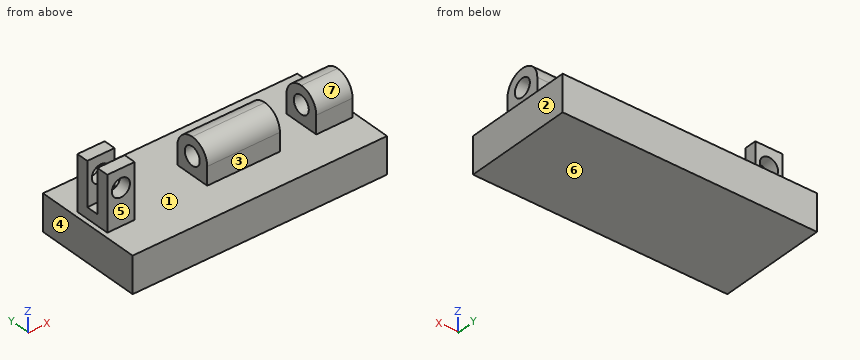
```python
from build123d import *

# Parameters (mm, degrees)
F0_W      = 177.8
F0_H      = 76.2
F1_DEPTH  = 25.4
F2_W      = 19.05
F2_H      = 38.1
F2_W_2    = 50.8
F2_H_2    = 25.4
F2_W_3    = 25.4
F3_DEPTH  = 25.4
F4_R      = 6.35
F5_DEPTH  = 101.6
F6_R      = 12.69999
F7_W      = 8.636
F7_H      = 30.48
F8_DEPTH  = 25.4
F9_R      = 6.35
F10_DEPTH = 25.4


# Not quite as in the source:
# - a fillet or chamfer is up to 0.001 mm smaller than in the source, because OpenCascade refuses the exact size


with BuildPart() as f1:
    # F0 (on Top) → F1 (new body)
    with BuildSketch(Plane.XY):
        with Locations((0, -12.7)):
            Rectangle(F0_W, F0_H)
    extrude(amount=F1_DEPTH)

    # F2 (on Front) → F3 (join)
    with BuildSketch(Plane.XZ):
        with Locations((-76.2, 44.45)):
            Rectangle(F2_W, F2_H)
        with Locations((9.525, 38.1)):
            Rectangle(F2_W_2, F2_H_2)
        with Locations((73.025, 38.1)):
            Rectangle(F2_W_3, F2_H_2)
    extrude(amount=F3_DEPTH)

    # F4 (on face) → F5 (cut, through all)
    with BuildSketch(Plane.YZ.offset(85.725)):
        with Locations((-12.7, 38.1)):
            Circle(F4_R)
    extrude(amount=-F5_DEPTH, mode=Mode.SUBTRACT)

    # F6 (radius 12.7 in the source; OpenCascade refuses exactly that, so slightly less here)
    f6_edges = [f1.edges().sort_by_distance(p)[0] for p in [
        (9.525, -25.4, 50.8),
        (9.525, 0, 50.8),
        (73.025, -25.4, 50.8),
        (73.025, 0, 50.8),
    ]]
    fillet(f6_edges, radius=F6_R)

    # F7 (on face) → F8 (cut)
    with BuildSketch(Plane(origin=(-85.725, 0, 0), x_dir=(0, -1, 0), z_dir=(-1, 0, 0))):
        with Locations((12.7, 48.26)):
            Rectangle(F7_W, F7_H)
    extrude(amount=-F8_DEPTH, mode=Mode.SUBTRACT)

    # F9 (on face) → F10 (cut)
    with BuildSketch(Plane.XZ.offset(25.4)):
        with Locations((-76.2, 50.8)):
            Circle(F9_R)
    extrude(amount=-F10_DEPTH, mode=Mode.SUBTRACT)


solid = f1.part
```
Geometry check sheet. Reference: the model listing, model coordinates, mm. Face numbers are marked on the shaded views. A direction names the side the tool comes from. Coordinates: 2 decimals unless noted, no trailing zeros. Order: outer loops, then holes, each group sorted by start corner. A loop starts at its lowest first (then second) coordinate and runs counter-clockwise, first axis right, second up. Notation, with made-up numbers: (-26.75, 51.25) - (16.25, 51.25) arc R19 cw to (16.25, 83.25) - close; hole circle Ø5 at (38.5, 88). An arc over 180 degrees is marked (long way). Answer as a JSON object with one key per item and string values. Group by question number.
Item 1: Sectioned sample at C-C, the plane y = -3.5. Record the cut outline in (x, z) (3 decimals), and give its area (3 significant figures).
Item 2: Sectioned sample at D-D, the plane z = 35. Record the cut outline in (x, y) (3 decimals), and give its area (3 significant figures).
Item 3: Sectioned sample at B-B, the plane x = -76.2. Record the cut outline in (y, z).
Item 4: Scan lines: probe 1 along Z at (x, y) = (72.5, -12.7); probe 2 along Z at (x, y) = (-76, -3); probe 3 along Y at (x, z) = (70, 38). Record each from-to range of solid material in increasing order.
Item 5: Depth check by flat-ended pin: pin 1 Ø6.5 at (x, z) = (7.5, 34) entering from -Y; pin 2 Ø1.5 at (x, y) = (49, -31.5) entering from -Z; pin 3 Ø7.5 at (y, z) = (-15, 40) entering from +X (3 decimals); pin 4 Ø23 at (x, y) = (-19, -15.5) entering from +Z. Enter the tip coordinate at first touch or a pass-through.
Item 6: Draft check along X on the marked faces 1, 2, 3 and 4. Enter one of: +X half, -X half, draft (parallel to the pull), parting line (faces both ways), or undercut.
Item 7: Tool access check on the marked faces 5, 6 and 7. Record the directions out of +Z, -Z, +X, -X, +Y, -Y that give a thin tool (end or side, any length) a straight path to the whole face; none if there is none.
Resolved:
{
 "1": {"outline": "(-88.9, 0) - (88.9, 0) - (88.9, 25.4) - (85.725, 25.4) - (85.725, 46.855) - (60.325, 46.855) - (60.325, 25.4) - (34.925, 25.4) - (34.925, 46.855) - (-15.875, 46.855) - (-15.875, 25.4) - (-66.675, 25.4) - (-66.675, 63.5) - (-85.725, 63.5) - (-85.725, 25.4) - (-88.9, 25.4) - close; hole circle Ø12.7 at (-76.2, 50.8)", "area": "6,750 mm^2"},
 "2": {"outline": "(-85.725, -25.4) - (-66.675, -25.4) - (-66.675, -17.018) - (-85.725, -17.018) - close; (-85.725, -8.382) - (-66.675, -8.382) - (-66.675, 0) - (-85.725, 0) - close; (-15.875, -25.4) - (34.925, -25.4) - (34.925, -18.242) - (-15.875, -18.242) - close; (-15.875, -7.158) - (34.925, -7.158) - (34.925, 0) - (-15.875, 0) - close; (60.325, -25.4) - (85.725, -25.4) - (85.725, -18.242) - (60.325, -18.242) - close; (60.325, -7.158) - (85.725, -7.158) - (85.725, 0) - (60.325, 0) - close", "area": "1,410 mm^2"},
 "3": {"outline": "(-50.8, 0) - (25.4, 0) - (25.4, 25.4) - (0, 25.4) - (0, 44.45) - (-8.38, 44.45) - (-8.38, 33.02) - (-17.02, 33.02) - (-17.02, 44.45) - (-25.4, 44.45) - (-25.4, 25.4) - (-50.8, 25.4) - close; (-25.4, 57.15) - (-17.02, 57.15) - (-17.02, 63.5) - (-25.4, 63.5) - close; (-8.38, 57.15) - (0, 57.15) - (0, 63.5) - (-8.38, 63.5) - close"},
 "4": {"probe 1": "0 to 31.75, 44.45 to 50.8", "probe 2": "0 to 44.45, 57.15 to 63.5", "probe 3": "-25.4 to -19.05, -6.35 to 0"},
 "5": {"pin 1": "y = -25.4", "pin 2": "z = 0", "pin 3": "x = 85.725", "pin 4": "z = 50.8"},
 "6": {"face 1": "undercut", "face 2": "+X half", "face 3": "draft", "face 4": "-X half"},
 "7": {"face 5": "+Z, +X, -X, -Y", "face 6": "-Z, +X, -X, +Y, -Y", "face 7": "+Z, +X, -Y"}
}
